Could you check a few things on this model? Use its own coordinates, in mm. A direction names the side the tool comes from. Give positions to 0.01 mm unless a question says otherwise; leave off trailing zeros. Loops run counter-clockwise (first coordinate to the right, second up) from the corner with the lowest first, then second, coordinate; pieces in that order, holes last. Notation, with made-up numbers: M 34,-15 L 82,-15 A21 cw 82,1 Z; hole C 15,-23 d2. An arc over 180 degrees is marked long. Return JSON: item names as keys, results as strings. Group by question number.
1. If we section it at D-D (z = -14): Write out the boundary of the cut face in (x, y) (3 decimals), plus the area to 3 significant figures.
2. Please list where these lines run through material, in increasing order: line 1 (Z direction, x = -8, y = 1); line 2 (X direction, y = 3, z = -1); line 3 (Z direction, x = -12.7, y = 3).
3. If we section it at A-A (z = 0): Write out the boundary of the cut face in (x, y) (1 decimal), plus the area to 3 significant figures.
4. If we section it at B-B (y = -7.5): Write out the boundary of the cut face in (x, z) (1 decimal), plus the area to 3 significant figures.
5. If we mould it in two halves opening along Z, with no side actions, what happens to faces 4 (the flat face through (-1, 0, -25.4)), 5 (the flat face through (13, 0, 25.4)), 6 (the cylindrical face through (-24, 0.7, 18.5)), 7 (the flat face through (38.1, 0, 0))? For each: +Z half, -Z half, draft (parallel to the pull), parting line (faces both ways), or undercut.
6. For faces 1 (the cylindrical face through (-4.67, 0.52, 18.99)), 2 (the flat face through (-11.112, 0, 23)), 3 (the flat face through (8, -9.525, 0)), which set-ups out of +Z, -Z, +X, -X, +Y, -Y let a thin tool reach every point of the face, with its end or its side?
7. If we section it at C-C (x = -16): Write out the boundary of the cut face in (y, z) (1 decimal).
8. For pin 1 (4 mm diameter, centred on y = -1.5, z = 21, fed in from -X); pin 2 (3 mm diameter, centred on y = 0, z = 20.64, fed in from -X), each with a flat end and sliding along its axis, tell me the tip position at first contact or that it passes through.
```python
from build123d import *

# Parameters (mm, degrees)
SKETCH1_W                                      = 76.2
SKETCH1_H                                      = 50.8
BOSS_EXTRUDE1_DEPTH                            = 9.525
SKETCH2_R                                      = 16.3195
CUT_EXTRUDE1_DEPTH                             = 50.595085442
SKETCH3_W                                      = 3.175
SKETCH3_H                                      = 28.019395236
CUT_EXTRUDE2_DEPTH                             = 50.595085442
CBORE_FOR_8_SOCKET_HEAD_CAP_SCREW1_D           = 4.4958
CBORE_FOR_8_SOCKET_HEAD_CAP_SCREW1_DEPTH       = 23.8125
CBORE_FOR_8_SOCKET_HEAD_CAP_SCREW1_CBORE_D     = 7.9375
CBORE_FOR_8_SOCKET_HEAD_CAP_SCREW1_CBORE_DEPTH = 4.1656
F_8_32_TAPPED_HOLE1_D                          = 3.4544
F_8_32_TAPPED_HOLE1_DEPTH                      = 12.7
F_8_32_TAPPED_HOLE1_TIP                        = 1.037806461
F_1_4_20_TAPPED_HOLE1_D                        = 5.1054


with BuildPart() as part:
    # Sketch1 → Boss-Extrude1 (new, symmetric)
    with BuildSketch(Plane(origin=(0, 0, 0), x_dir=(1, 0, 0), z_dir=(0, 1, 0))):
        Rectangle(SKETCH1_W, SKETCH1_H)
    extrude(amount=BOSS_EXTRUDE1_DEPTH, both=True)

    # Sketch2 → Cut-Extrude1 (cut, through all)
    with BuildSketch(Plane(origin=(0, 9.525, 0), x_dir=(1, 0, 0), z_dir=(0, 1, 0))):
        with Locations(Location((-12.7, 0, 0), (0, 0, 270))):
            Circle(SKETCH2_R)
    extrude(amount=-CUT_EXTRUDE1_DEPTH, mode=Mode.SUBTRACT)

    # Sketch3 → Cut-Extrude2 (cut, through all)
    with BuildSketch(Plane(origin=(0, 9.525, 0), x_dir=(1, 0, 0), z_dir=(0, 1, 0))):
        with Locations((-12.7, -14.009697618)):
            Rectangle(SKETCH3_W, SKETCH3_H)
    extrude(amount=-CUT_EXTRUDE2_DEPTH, mode=Mode.SUBTRACT)

    # CBORE for #8 Socket Head Cap Screw1
    with Locations(Plane.ZY.offset(38.1)):
        with Locations((20.6375, 0)):
            CounterBoreHole(CBORE_FOR_8_SOCKET_HEAD_CAP_SCREW1_D / 2, CBORE_FOR_8_SOCKET_HEAD_CAP_SCREW1_CBORE_D / 2, CBORE_FOR_8_SOCKET_HEAD_CAP_SCREW1_CBORE_DEPTH, depth=CBORE_FOR_8_SOCKET_HEAD_CAP_SCREW1_DEPTH)

    # #8-32 Tapped Hole1
    with Locations(Plane.ZY.offset(11.1125)):
        with Locations((20.6375, 0)):
            Hole(F_8_32_TAPPED_HOLE1_D / 2, depth=F_8_32_TAPPED_HOLE1_DEPTH)
            with Locations((0, 0, -(F_8_32_TAPPED_HOLE1_DEPTH + F_8_32_TAPPED_HOLE1_TIP / 2))):  # 118° drill point
                Cone(0, F_8_32_TAPPED_HOLE1_D / 2, F_8_32_TAPPED_HOLE1_TIP, mode=Mode.SUBTRACT)

    # 1/4-20 Tapped Hole1 (through all)
    with Locations(Plane(origin=(0, 9.525, 0), x_dir=(1, 0, 0), z_dir=(0, 1, 0))):
        with Locations((28.575, 0)):
            Hole(F_1_4_20_TAPPED_HOLE1_D / 2)


solid = part.part
```
Answer:
{
 "1": {"outline": "M -38.1,-9.525 L -21.086,-9.525 L -21.086,9.525 L -38.1,9.525 Z; M -4.314,-9.525 L 38.1,-9.525 L 38.1,9.525 L -4.314,9.525 Z", "area": "1,130 mm²"},
 "2": {"line 1": "z = -25.4 to -15.63, 15.63 to 19.23, 22.05 to 25.4", "line 2": "x = -38.1 to -28.99, 3.59 to 26.23, 30.92 to 38.1", "line 3": "z = -25.4 to -16.32"},
 "3": {"outline": "M -38.1,-9.5 L -29,-9.5 L -29,9.5 L -38.1,9.5 Z; M 3.6,-9.5 L 26,-9.5 L 26,9.5 L 3.6,9.5 Z; M 31.1,-9.5 L 38.1,-9.5 L 38.1,9.5 L 31.1,9.5 Z", "area": "733 mm²"},
 "4": {"outline": "M -38.1,-25.4 L 38.1,-25.4 L 38.1,25.4 L -11.1,25.4 L -11.1,16.2 A16.3 cw long -14.3,16.2 L -14.3,25.4 L -38.1,25.4 Z; hole C 28.6,0 d5.1", "area": "2,980 mm²"},
 "5": {"face 4": "-Z half", "face 5": "+Z half", "face 6": "undercut", "face 7": "draft"},
 "6": {"face 1": "-X", "face 2": "+Z, +Y, -Y", "face 3": "+Z, -Z, +X, -X, -Y"},
 "7": {"outline": "M -9.5,-25.4 L 9.5,-25.4 L 9.5,-16 L -9.5,-16 Z; M -9.5,16 L 9.5,16 L 9.5,25.4 L -9.5,25.4 Z; hole C 0,20.6 d4.5"},
 "8": {"pin 1": "stops at x = -33.93", "pin 2": "stops at x = 1.72"}
}
